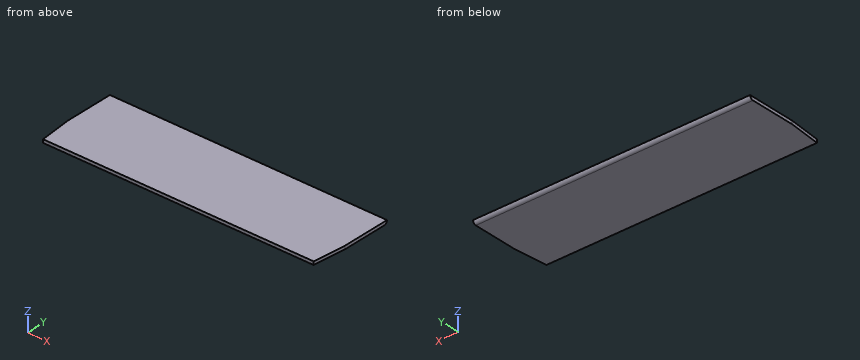
from build123d import *

# Parameters (mm, degrees)
F1_DEPTH = 2
F3_DEPTH = 170


with BuildPart() as f1:
    # F0 (on Top) → F1 (new body)
    with BuildSketch(Plane.XY):
        Polygon((84.566931, 0.678322), (-85.433069, 0.678322), (-85.433069, -27.321678), (-83.433069, -47.321678), (82.566931, -47.321678), (84.566931, -27.321678), align=None)
    extrude(amount=F1_DEPTH)

    # F2 (on face) → F3 (join)
    with BuildSketch(Plane.YZ.offset(84.566931)):
        with BuildLine():
            Line((0.678322, 2), (0.678322, 0))
            ThreePointArc((0.678322, 0), (2.092536, 0.585786), (2.678322, 2))
            Line((2.678322, 2), (0.678322, 2))
        make_face()
    extrude(amount=-F3_DEPTH)


solid = f1.part
The listing builds one solid part. Answer for the finished solid, in the listing's coordinates (mm). Round coordinates to 2 decimals unless told otherwise and drop trailing zeros. Loops run counter-clockwise (first coordinate to the right, second up) from the corner with the lowest first, then second, coordinate; pieces in that order, holes last. Notation, with made-up numbers: M 77,37.25 L 115,37.25 A33 ccw 115,76.25 Z; hole C 18.25,56 d11. An arc over 180 degrees is marked long. Write each question's results on one line, items separated by ' | '. Start each with the question number.
1) Find section B-B on y = -40.5. Write down the section's boundary in (x, z), plus the area to 3 significant figures.
2) Straight lines are drawn through the part: probe 1 along X at (y, z) = (-27.5, 0.1); probe 2 along Y at (x, z) = (-42, 1.85); probe 3 along Y at (x, z) = (24.5, 0.5). For each, find the intervals that lie inside material, in ascending order.
3) Find section A-A on z = 0.45. Write down the section's boundary in (x, y), plus the area to 3 significant figures.
Final values:
1) outline: M -84.12,0 L 83.25,0 L 83.25,2 L -84.12,2 Z | area: 335 mm²
2) probe 1: -85.42 to 84.55 | probe 2: -47.32 to 2.67 | probe 3: -47.32 to 2
3) outline: M -85.43,-27.32 L -83.43,-47.32 L 82.57,-47.32 L 84.57,-27.32 L 84.57,1.94 L -85.43,1.94 Z | area: 8,330 mm²
